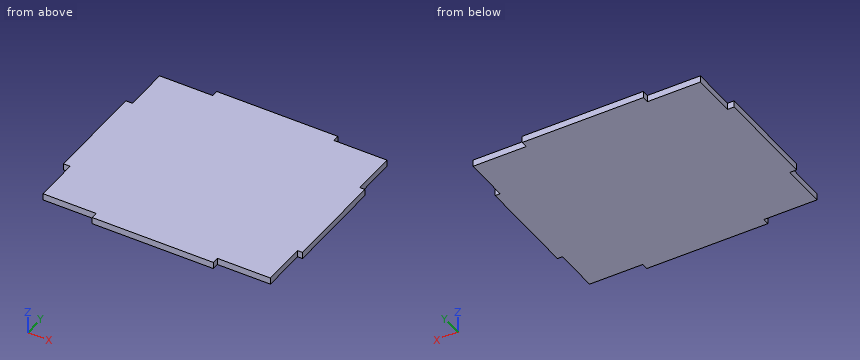
from build123d import *

# Parameters (mm, degrees)
SKETCH_1_W          = 72
SKETCH_1_H          = 62
EXTRUDE_1_DEPTH     = 2
SKETCH_2_W          = 2
SKETCH_2_H          = 15.5
CUT_EXTRUDE_1_DEPTH = 3
SKETCH_3_W          = 18
SKETCH_3_H          = 2
CUT_EXTRUDE_2_DEPTH = 3


with BuildPart() as part:
    # ｽｹｯﾁ1 → ﾎﾞｽ - 押し出し1 (new body)
    with BuildSketch(Plane.XY):
        with Locations((-1.042641223, 9.736263736)):
            Rectangle(SKETCH_1_W, SKETCH_1_H)
    extrude(amount=EXTRUDE_1_DEPTH)

    # ｽｹｯﾁ2 → ｶｯﾄ - 押し出し1 (cut, through all)
    with BuildSketch(Plane.XY.offset(2)):
        with Locations((34.457358777, -13.513736264)):
            Rectangle(SKETCH_2_W, SKETCH_2_H)
        with Locations((34.457358777, 32.986263736)):
            Rectangle(SKETCH_2_W, SKETCH_2_H)
        with Locations((-36.042641223, 32.986263736)):
            Rectangle(SKETCH_2_W, SKETCH_2_H)
        with Locations((-36.042641223, -13.513736264)):
            Rectangle(SKETCH_2_W, SKETCH_2_H)
    extrude(amount=-CUT_EXTRUDE_1_DEPTH, mode=Mode.SUBTRACT)

    # ｽｹｯﾁ3 → ｶｯﾄ - 押し出し2 (cut, through all)
    with BuildSketch(Plane.XY.offset(2)):
        with Locations((-28.042641223, 39.736263736)):
            Rectangle(SKETCH_3_W, SKETCH_3_H)
        with Locations((26.457358777, 39.736263736)):
            Rectangle(SKETCH_3_W, SKETCH_3_H)
        with Locations((-28.042641223, -20.263736264)):
            Rectangle(SKETCH_3_W, SKETCH_3_H)
        with Locations((26.457358777, -20.263736264)):
            Rectangle(SKETCH_3_W, SKETCH_3_H)
    extrude(amount=-CUT_EXTRUDE_2_DEPTH, mode=Mode.SUBTRACT)


solid = part.part
Work out the finished part from the listing and answer in its coordinate system (mm). Round coordinates to 2 decimals unless told otherwise and drop trailing zeros. Loops run counter-clockwise (first coordinate to the right, second up) from the corner with the lowest first, then second, coordinate; pieces in that order, holes last. Notation, with made-up numbers: (0.5, -4) - (47.5, -4) arc R31 ccw to (47.5, 33) - close; hole circle Ø5 at (56.25, 23.25). An arc over 180 degrees is marked (long way). Use one line per item in the form item = value. Start each with the question number.
(1) Find section C-C on y = -17. Determine the outline of the cut face in (x, z), and give its area (3 significant figures).
(2) Flat-ended cylindrical pins translate along their axes: P1, Ø0.6, axis at y = 40, z = 0.5, coming from the +X side; P2, Ø0.6, axis at y = -14, z = 1, coming from the +X side; P3, Ø0.6, axis at x = -24, z = 1, coming from the -Y side. Find the tip coordinate at first contact, or state that the pin passes through.
(3) Find section B-B on x = 26.5. Determine the outline of the cut face in (y, z).
(4) Consider line 1 (Y direction, x = 21, z = 1.4); line 2 (X direction, y = 29, z = 1.75). Determine where each line is inside the solid, lowest interval first.
(5) Find section A-A on z = 1.6. Determine the outline of the cut face in (x, y), and give its area (3 significant figures).
Answer list:
q1.outline = (-35.04, 0) - (33.46, 0) - (33.46, 2) - (-35.04, 2) - close
q1.area = 137 mm^2
q2.P1 = 17.46
q2.P2 = 33.46
q2.P3 = -19.26
q3.outline = (-19.26, 0) - (38.74, 0) - (38.74, 2) - (-19.26, 2) - close
q4.line_1 = -19.26 to 38.74
q4.line_2 = -35.04 to 33.46
q5.outline = (-37.04, -5.76) - (-35.04, -5.76) - (-35.04, -19.26) - (-19.04, -19.26) - (-19.04, -21.26) - (17.46, -21.26) - (17.46, -19.26) - (33.46, -19.26) - (33.46, -5.76) - (34.96, -5.76) - (34.96, 25.24) - (33.46, 25.24) - (33.46, 38.74) - (17.46, 38.74) - (17.46, 40.74) - (-19.04, 40.74) - (-19.04, 38.74) - (-35.04, 38.74) - (-35.04, 25.24) - (-37.04, 25.24) - close
q5.area = 4,230 mm^2
